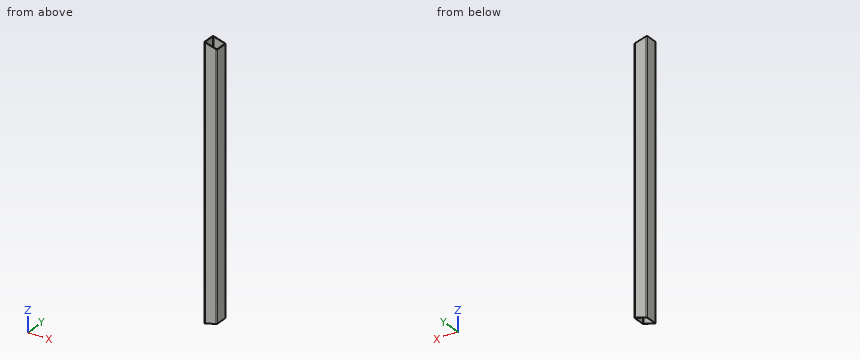
Autodesk Inventor part; units mm, degrees
ref_plane "YZ Plane" through (0, 0, 0) normal (1, 0, 0) x (0, 1, 0)
ref_plane "XZ Plane" through (0, 0, 0) normal (0, 1, 0) x (-1, 0, 0)
ref_plane "XY Plane" through (0, 0, 0) normal (0, 0, 1) x (1, 0, 0)
sketch "Sketch1" plane through (0, 0, 0) normal (0, 0, 1) x (1, 0, 0)
  line L0 (-60, -52) -> (-60, 52)
  line L1 (-52, 60) -> (52, 60)
  line L2 (60, 52) -> (60, -52)
  line L3 (52, -60) -> (-52, -60)
  arc A0 (-60, -52) -> (-52, -60) centre (-52, -52) ccw
  arc A1 (60, 52) -> (52, 60) centre (52, 52) ccw
  arc A2 (-52, 60) -> (-60, 52) centre (-52, 52) ccw
  arc A3 (52, -60) -> (60, -52) centre (52, -52) ccw
  arc A4 (-52, 56) -> (-56, 52) centre (-52, 52) ccw
  line L4 (-52, 56) -> (52, 56)
  arc A5 (56, 52) -> (52, 56) centre (52, 52) ccw
  line L5 (56, 52) -> (56, -52)
  arc A6 (52, -56) -> (56, -52) centre (52, -52) ccw
  line L6 (52, -56) -> (-52, -56)
  arc A7 (-56, -52) -> (-52, -56) centre (-52, -52) ccw
  line L7 (-56, -52) -> (-56, 52)
  point P0 (0, 0)
  point P1 (0, 0)
  point P2 (0, 60)
  point P3 (60, 0)
  dimension "d0" = 8
  dimension "d1" = 120
  dimension "d2" = 120
  dimension "d3" = 4
extrude "Extrusion1" add sketch "Sketch1" along normal mid plane 2500
sketch "Sketch2" plane through (-52, -60, 1250) normal (0, -1, 0) x (1, 0, 0)
  line L0 (-8, -2500) -> (-8, 0)
  line L1 (-8, 0) -> (112, -32.1539)
  line L2 (112, -2500) -> (112, 0)
  line L3 (0, 0) -> (104, 0)
  line L4 (112, 0) -> (104, 0)
  line L5 (0, 0) -> (-8, 0)
  point P0 (52, -1250)
  dimension "d16" = 15
extrude "Extrusion2" cut sketch "Sketch2" against normal blind 2000
mirror "Mirror1" about plane through (0, 0, 0) normal (0, 0, 1) of "Extrusion2"
equation "\"d0\" = d6"
equation "\"d1\" = d7"
equation "\"d2\" = d8"
equation "\"d3\" = d9"
equation "\"d6\" = 8"
equation "\"d7\" = 120"
equation "\"d8\" = 120"
equation "\"d9\" = 4"
properties part number "Crossbar"
Could you check a few things on this model? Use its own coordinates, in mm. Coordinates: 2 decimals unless noted, no trailing zeros. Loops run counter-clockwise (first coordinate to the right, second up) from the corner with the lowest first, then second, coordinate; pieces in that order, holes last.
1) Imagine slicing it at C-C (x = -11.5). List the corners of the cut face in (y, z) for me.
Reported:
outline: (-60, -1237) - (-56, -1237) - (-56, 1237) - (-60, 1237) - close; (56, -1237) - (60, -1237) - (60, 1237) - (56, 1237) - close
2) Imagine slicing it at B-B (z = 210). List the corners of the cut face in (x, y) for me, and give its area (3 significant figures).
Reported:
outline: (-60, -52) arc R8 ccw to (-52, -60) - (52, -60) arc R8 ccw to (60, -52) - (60, 52) arc R8 ccw to (52, 60) - (-52, 60) arc R8 ccw to (-60, 52) - close; hole (-56, -52) arc R4 ccw to (-52, -56) - (52, -56) arc R4 ccw to (56, -52) - (56, 52) arc R4 ccw to (52, 56) - (-52, 56) arc R4 ccw to (-56, 52) - close
area: 1,810 mm2
3) Imagine slicing it at A-A (y = 5.5). List the corners of the cut face in (x, z) for me, and give its area (3 significant figures).
Reported:
outline: (-60, -1250) - (-56, -1248.93) - (-56, 1248.93) - (-60, 1250) - close; (56, -1218.92) - (60, -1217.85) - (60, 1217.85) - (56, 1218.92) - close
area: 19,700 mm2
4) Please list where these lines run through material, in increasing order: line 1 along X through (y, z) = (-50.5, 608); line 2 along X through (y, z) = (-53.5, -305).
Reported:
line 1: x = -60 to -56, 56 to 60
line 2: x = -59.86 to -55.71, 55.71 to 59.86
